```python
from build123d import *
from build123d.topology import SkipClean

# Parameters (mm, degrees)
CUT_EXTRUDE1_DEPTH      = 6.196152423
CUT_EXTRUDE1_DEPTH_BACK = 6.196152423
SKETCH2_R               = 0.75
CUT_EXTRUDE2_DEPTH      = 6.141741007
CUT_EXTRUDE2_DEPTH_BACK = 6.141741007
SKETCH3_R               = 0.75


with BuildPart() as part:
    # Sketch1 → Revolve1 (revolve)
    with SkipClean():  # the faces are left unmerged after this step: merging them gives an invalid solid
        with BuildSketch(Plane.XY):
            with BuildLine():
                ThreePointArc((3, 0), (2.121320344, 2.121320344), (0, 3))
                Line((0, 3), (0, -3))
                ThreePointArc((0, -3), (2.121320344, -2.121320344), (3, 0))
            make_face()
            with BuildLine():
                Line((0, -3), (0, 3))
                ThreePointArc((0, 3), (-3, 0), (0, -3))
            make_face()
        revolve(axis=Axis((0, 3, 0), (0, -1, 0)))

    # Sketch2 → Cut-Extrude1 (cut, two sides: drawn at the far end of the back side and taken through both)
    with SkipClean():  # the faces are left unmerged after this step: merging them gives an invalid solid
        with BuildSketch(Plane(origin=(0, 0, 0), x_dir=(0, 0, -1), z_dir=(1, 0, 0)).offset(-CUT_EXTRUDE1_DEPTH_BACK)):
            Circle(SKETCH2_R)
        extrude(amount=CUT_EXTRUDE1_DEPTH + CUT_EXTRUDE1_DEPTH_BACK, mode=Mode.SUBTRACT)

    # Sketch3 → Cut-Extrude2 (cut, two sides: drawn at the far end of the back side and taken through both)
    with SkipClean():  # the faces are left unmerged after this step: merging them gives an invalid solid
        with BuildSketch(Plane.XY.offset(-CUT_EXTRUDE2_DEPTH_BACK)):
            with Locations(Location((0, 0, 0), (0, 0, 270))):
                Circle(SKETCH3_R)
        extrude(amount=CUT_EXTRUDE2_DEPTH + CUT_EXTRUDE2_DEPTH_BACK, mode=Mode.SUBTRACT)


solid = part.part
```
The model under review builds one solid part; all positions refer to its coordinate system, in mm. Give positions to 0.01 mm unless a question says otherwise; leave off trailing zeros. Loops run counter-clockwise (first coordinate to the right, second up) from the corner with the lowest first, then second, coordinate; pieces in that order, holes last. Notation, with made-up numbers: (33, 82) - (58, 82) arc R3 ccw to (58, 86) - close; hole circle Ø11 at (63.5, 2). An arc over 180 degrees is marked (long way). Answer as a JSON object with one key per item and string values.
Q1. To check wall thickness, follow line 1 along Z through (x, y) = (-1.2, 0); line 2 along Y through (x, z) = (1.3, 0); line 3 along Y through (x, z) = (-0.6, 1.9). State the ranges of each line that lie inside material, in increasing order.
Worked out:
{"line 1": "z = -2.75 to -0.75, 0.75 to 2.75", "line 2": "y = -2.7 to -0.75, 0.75 to 2.7", "line 3": "y = -2.24 to -0.45, 0.45 to 2.24"}
Q2. Add section C-C on x = 0.4. State the section outline as (y, z) points, plus the area to 3 significant figures.
Worked out:
{"outline": "(-0.63, -2.9) - (-0.63, -0.4) arc R0.75 cw to (-0.63, 0.4) - (-0.63, 2.9) arc R2.97 ccw to start; (0.63, -2.9) arc R2.97 ccw to (0.63, 2.9) - (0.63, 0.4) arc R0.75 cw to (0.63, -0.4) - close", "area": "20.2 mm^2"}
Q3. Insertion check: pin 1 (3 mm diameter, centred on x = -2, y = 0.5, fed in from -Z); pin 2 (1 mm diameter, centred on x = -1, z = -2, fed in from -Y); pin 3 (1 mm diameter, centred on x = 2.5, y = -0.5, fed in from +Z); pin 4 (1 mm diameter, centred on x = -0.5, z = 0.5, fed in from -Y). Each pin has a flat end and moves straight along its axis. Give the tip position at first contact, or say it passes through.
Worked out:
{"pin 1": "stops at z = -2.9", "pin 2": "stops at y = -2.45", "pin 3": "stops at z = 2.19", "pin 4": "stops at y = -2.99"}
Q4. Mouldability with a two-part tool opening along Z and no side actions: class faces 1 (the cylindrical face through (-0.456, 0.595, -1.795)), 2 (the cylindrical face through (-1.8, -0.29, -0.69)) as +Z half, -Z half, draft (parallel to the pull), parting line (faces both ways), or undercut.
Worked out:
{"face 1": "draft", "face 2": "undercut"}
Q5. Add section D-D on z = 1.7. State the section outline as (x, y) points, plus the area to 3 significant figures.
Worked out:
{"outline": "circle Ø4.94 at (0, 0); hole circle Ø1.5 at (0, 0)", "area": "17.4 mm^2"}
Q6. Add section A-A on y = 0. State the section outline as (x, z) points, plus the area to 3 significant figures.
Worked out:
{"outline": "(-2.9, -0.75) arc R3 ccw to (-0.75, -2.9) - (-0.75, -0.75) - close; (-2.9, 0.75) - (-0.75, 0.75) - (-0.75, 2.9) arc R3 ccw to start; (0.75, -2.9) arc R3 ccw to (2.9, -0.75) - (0.75, -0.75) - close; (0.75, 0.75) - (2.9, 0.75) arc R3 ccw to (0.75, 2.9) - close", "area": "12.7 mm^2"}
